Verification items for the finished model (mm, model axes). A direction names the side the tool comes from. Coordinates: 2 decimals unless noted, no trailing zeros. Write each loop counter-clockwise with the first axis right and the second up, starting at its lowest first coordinate (ties: lowest second). Pieces come first, ordered by that corner, then holes. Notation, with made-up numbers: (37.25, 8) -> (43.25, 8) arc R19 cw to (43.25, 21) -> close; hole circle Ø3 at (-1, -15.5). An arc over 180 degrees is marked (long way). Use a Markdown table: item, result. Add a question column.
from build123d import *

# Parameters (mm, degrees)
SKETCH1_R           = 12.5
BOSS_EXTRUDE1_DEPTH = 15
SKETCH2_OUTSIDE_W   = 78.684
SKETCH2_OUTSIDE_H   = 58.684
CUT_EXTRUDE1_DEPTH  = 37.5
SKETCH3_R           = 12.5
BOSS_EXTRUDE2_DEPTH = 25
FILLET1_R           = 2


with BuildPart() as part:
    # Sketch1 → Boss-Extrude1 (new, symmetric)
    with BuildSketch(Plane(origin=(0, 0, 0), x_dir=(1, 0, 0), z_dir=(0, 1, 0))):
        with BuildLine():
            Line((-29.664793948, 15), (-95, 15))
            Line((-95, 15), (-95, -15))
            Line((-95, -15), (-29.664793948, -15))
            ThreePointArc((-29.664793948, -15), (-21.998275168, -16.257430009), (-15.135098953, -19.897959184))
            ThreePointArc((-15.135098953, -19.897959184), (25, 0), (-15.135098953, 19.897959184))
            ThreePointArc((-15.135098953, 19.897959184), (-21.998275168, 16.257430009), (-29.664793948, 15))
        make_face()
        with Locations(Location((0, 0, 0), (0, 0, 270))):
            Circle(SKETCH1_R, mode=Mode.SUBTRACT)
    extrude(amount=BOSS_EXTRUDE1_DEPTH, both=True)

    # Sketch2 outside → Cut-Extrude1 (cut)
    with BuildSketch(Plane.ZY.offset(95)):
        Rectangle(SKETCH2_OUTSIDE_W, SKETCH2_OUTSIDE_H)
        Polygon((6.213203436, 15), (-6.213203436, 15), (-15, 6.213203436), (-15, -6.213203436), (-6.213203436, -15), (6.213203436, -15), (15, -6.213203436), (15, 6.213203436), align=None, mode=Mode.SUBTRACT)
    extrude(amount=-CUT_EXTRUDE1_DEPTH, mode=Mode.SUBTRACT)

    # Sketch3 → Boss-Extrude2 (add)
    with BuildSketch(Plane.ZY.offset(95)):
        Circle(SKETCH3_R)
    extrude(amount=BOSS_EXTRUDE2_DEPTH)

    # Fillet1
    fillet1_edges = [part.edges().sort_by_distance(p)[0] for p in [
        (-57.5, 10.606601718, -10.606601718),
        (-57.5, -10.606601718, -10.606601718),
        (-57.5, 10.606601718, 10.606601718),
        (-57.5, -10.606601718, 10.606601718),
    ]]
    fillet(fillet1_edges, radius=FILLET1_R)

    # Sketch4 → Cut-Revolve1 (revolve, cut)
    with BuildSketch(Plane.XY):
        Polygon((-95, 15), (-95, 27.0023011), (-88.070468229, 27.0023011), align=None)
    revolve(axis=Axis((0, 0, 0), (-1, 0, 0)), mode=Mode.SUBTRACT)


solid = part.part
1) Cross-section at A-A on x = 0. Record the boundary of the cut face in (y, z), then the cut area to 3 significant figures.
2) Cross-section at B-B on x = -61. Record the boundary of the cut face in (y, z), then the cut area to 3 significant figures.
3) Cross-section at D-D on x = -103. Record the boundary of the cut face in (y, z), then the cut area to 3 significant figures.
4) Set-up check for faces 4 (the face through (-77.498, 10.545, 10.668)), 5 (the face through (-57.5, -13, 13)), 6 (the face through (-57.5, -13, -13)), 7 (the face through (-57.5, 13, -13)): record each of +Z, -Z, +X, -X, +Y, -Y from which the full face is reachable in a straight line by a thin tool's end or side.
5) Cross-section at C-C on z = 22. Record the boundary of the cut face in (x, y).
6) Gauge pin test, flat ends, axial feed: pin 1 (8 mm diameter, centred on y = -1.5, z = -10, fed in from +X); pin 2 (5 mm diameter, centred on x = -95, y = -11.5, fed in from +Z); pin 3 (22.5 mm diameter, centred on x = 0, z = 0, fed in from +Y); pin 4 (3 mm diameter, centred on x = -3.5, z = 10.5, fed in from +Y). Record the tip position at first contact, or that the pin passes through.
7) Release check for a two-part mould opening along X. For faces 1 (the face through (-57.5, 13, 13)), 2 (the face through (3.755, -0.21, 11.923)), 3 (the face through (-77.498, -10.668, 10.545)) record: released by +X, released by -X, zero draft, split by the parting line, or undercut.
8) Thickness scan on L1, parallel to X at y = 6, z = 0; L2, parallel to X at y = 5.5, z = 10; L3, parallel to Z at x = -93.5, y = 1. Record the ranges inside material, lowest first.
Returned:
| question | item | result |
|---|---|---|
| 1 | outline | (-15, -25) -> (15, -25) -> (15, -12.5) -> (-15, -12.5) -> close; (-15, 12.5) -> (15, 12.5) -> (15, 25) -> (-15, 25) -> close |
| 1 | area | 750 mm² |
| 2 | outline | (-15, -6.21) -> (-6.21, -15) -> (6.21, -15) -> (15, -6.21) -> (15, 6.21) -> (6.21, 15) -> (-6.21, 15) -> (-15, 6.21) -> close |
| 2 | area | 746 mm² |
| 3 | outline | circle Ø25 at (0, 0) |
| 3 | area | 491 mm² |
| 4 | face 4 | +Z, -X, +Y |
| 4 | face 5 | +Z, -X, -Y |
| 4 | face 6 | -Z, -X, -Y |
| 4 | face 7 | -Z, -X, +Y |
| 5 | outline | (-11.87, -15) -> (11.87, -15) -> (11.87, 15) -> (-11.87, 15) -> close |
| 6 | pin 1 | stops at x = 24.27 |
| 6 | pin 2 | stops at z = 12.21 |
| 6 | pin 3 | passes through |
| 6 | pin 4 | stops at y = 15 |
| 7 | face 1 | released by -X |
| 7 | face 2 | undercut |
| 7 | face 3 | zero draft |
| 8 | L1 | x = -120 to -12.5, 12.5 to 25 |
| 8 | L2 | x = -120 to -7.5, 7.5 to 22.91 |
| 8 | L3 | z = -15 to 15 |
